from build123d import *

# Parameters (mm, degrees)
F0_W     = 2.35
F0_H     = 1.5
F1_DEPTH = 2.1
F2_START = -2.1
F0_R     = 2.8
F2_DEPTH = 0.9


with BuildPart() as f1:
    # F0 (on Right) → F1 (new body, symmetric)
    with BuildSketch(Plane.YZ):
        with BuildLine():
            Line((-3.65, 1.5), (-3.65, 2.1073284825))
            Line((-3.65, 2.1073284825), (0, 4.2146569651))
            Line((0, 4.2146569651), (3.65, 2.1073284825))
            Line((3.65, 2.1073284825), (3.65, -2.1073284825))
            Line((3.65, -2.1073284825), (0, -4.2146569651))
            Line((0, -4.2146569651), (-3.65, -2.1073284825))
            Line((-3.65, -2.1073284825), (-3.65, -1.5))
            Line((-3.65, -1.5), (-6, -1.5))
            Line((-6, -1.5), (-6, -5))
            Line((-6, -5), (6, -5))
            Line((6, -5), (6, 0))
            ThreePointArc((6, 0), (4.2426406871, 4.2426406871), (0, 6))
            ThreePointArc((0, 6), (-3.6742346142, 4.7434164903), (-5.8094750193, 1.5))
            Line((-5.8094750193, 1.5), (-3.65, 1.5))
        make_face()
        with Locations((-4.825, -0.75)):
            Rectangle(F0_W, F0_H)
        with BuildLine():
            Line((-3.65, 0), (-3.65, 1.5))
            Line((-3.65, 1.5), (-5.8094750193, 1.5))
            ThreePointArc((-5.8094750193, 1.5), (-5.9521781776, 0.7560257549), (-6, 0))
            Line((-6, 0), (-3.65, 0))
        make_face()
    extrude(amount=F1_DEPTH, both=True)

    # F0 (on Right) → F2 (join)
    with BuildSketch(Plane.YZ.offset(F2_START)):
        with BuildLine():
            Line((-3.65, 0), (-3.65, 1.5))
            Line((-3.65, 1.5), (-5.8094750193, 1.5))
            ThreePointArc((-5.8094750193, 1.5), (-5.9521781776, 0.7560257549), (-6, 0))
            Line((-6, 0), (-3.65, 0))
        make_face()
        with Locations((-4.825, -0.75)):
            Rectangle(F0_W, F0_H)
        with BuildLine():
            Line((-3.65, 1.5), (-3.65, 2.1073284825))
            Line((-3.65, 2.1073284825), (0, 4.2146569651))
            Line((0, 4.2146569651), (3.65, 2.1073284825))
            Line((3.65, 2.1073284825), (3.65, -2.1073284825))
            Line((3.65, -2.1073284825), (0, -4.2146569651))
            Line((0, -4.2146569651), (-3.65, -2.1073284825))
            Line((-3.65, -2.1073284825), (-3.65, -1.5))
            Line((-3.65, -1.5), (-6, -1.5))
            Line((-6, -1.5), (-6, -5))
            Line((-6, -5), (6, -5))
            Line((6, -5), (6, 0))
            ThreePointArc((6, 0), (4.2426406871, 4.2426406871), (0, 6))
            ThreePointArc((0, 6), (-3.6742346142, 4.7434164903), (-5.8094750193, 1.5))
            Line((-5.8094750193, 1.5), (-3.65, 1.5))
        make_face()
        Polygon((0, 4.2146569651), (-3.65, 2.1073284825), (-3.65, 1.5), (-3.65, 0), (-3.65, -1.5), (-3.65, -2.1073284825), (0, -4.2146569651), (3.65, -2.1073284825), (3.65, 2.1073284825), align=None)
        Circle(F0_R, mode=Mode.SUBTRACT)
    extrude(amount=-F2_DEPTH)

    # F0 (on Right) → F3 (revolve)
    with BuildSketch(Plane.YZ):
        with BuildLine():
            ThreePointArc((-6, 0), (-5.9521781776, 0.7560257549), (-5.8094750193, 1.5))
            Line((-5.8094750193, 1.5), (-13.15, 1.5))
            Line((-13.15, 1.5), (-13.15, 0))
            Line((-13.15, 0), (-6, 0))
        make_face()
        with BuildLine():
            Line((-3.65, 0), (-3.65, 1.5))
            Line((-3.65, 1.5), (-5.8094750193, 1.5))
            ThreePointArc((-5.8094750193, 1.5), (-5.9521781776, 0.7560257549), (-6, 0))
            Line((-6, 0), (-3.65, 0))
        make_face()
    revolve(axis=Axis((0, -8.4, 0), (0, 1, 0)))

    # F4: F1 across plane


with BuildPart() as f1_1:
    add(f1.part)
    add(f1.part.mirror(Plane.YZ))


solid = f1_1.part
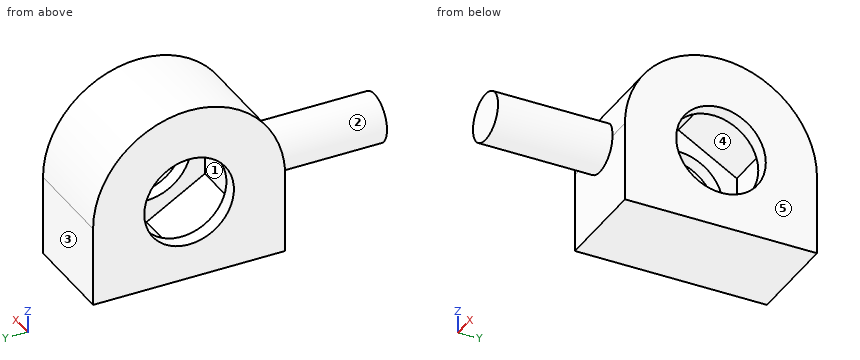
For this review, take the finished solid that the model builds, in its own axes (mm). Face numbers are marked on the shaded views. A direction names the side the tool comes from. Give positions to 0.01 mm unless a question says otherwise; leave off trailing zeros. Loops run counter-clockwise (first coordinate to the right, second up) from the corner with the lowest first, then second, coordinate; pieces in that order, holes last.
Item 1: Draft analysis for pull direction Y (two halves, no side actions). For the marked faces 1, 2 and 3, state which applies: +Y half, -Y half, draft (parallel to the pull), parting line (faces both ways), or undercut.
Item 2: For line 1 along Z through (x, y) = (2.8, 0); line 2 along X through (y, z) = (-2, 2); line 3 along Z through (x, y) = (0, -10.5), list the stretches that pass through material, from the lowest coordinate up.
Item 3: Take a section at B-B, the plane x = 0. State the section outline as (y, z) points.
Item 4: Take a section at D-D, the plane z = 4. State the section outline as (x, y) points.
Item 5: Take a section at C-C, the plane z = -2.5. State the section outline as (x, y) points, and give its area (3 significant figures).
Item 6: Take a section at A-A, the plane y = 1. State the section outline as (x, z) points, and give its area (3 significant figures).
Item 7: Tool access review of the marked faces 4 and 5: name each direction out of +Z, -Z, +X, -X, +Y, -Y from which nothing blocks a thin tool from reaching the whole face with its end or side.
Item 8: Insertion check: pin 1 (1 mm diameter, centred on x = -1, z = 5, fed in from +Y). The pin has a flat end and moves straight along its axis. Give the tip position at first contact, or say it passes through.
Calculated:
1. face 1: undercut
1. face 2: draft
1. face 3: +Y half
2. line 1: z = -5 to -2.8, 2.8 to 6
2. line 2: x = -3 to -2.1, 2.1 to 3
2. line 3: z = -1.5 to 1.5
3. outline: (-13.15, -1.5) - (-6, -1.5) - (-6, -5) - (6, -5) - (6, 0) arc R6 ccw to (-5.81, 1.5) - (-13.15, 1.5) - close; hole (-3.65, -2.11) - (0, -4.21) - (3.65, -2.11) - (3.65, 2.11) - (0, 4.21) - (-3.65, 2.11) - close
4. outline: (-3, -4.47) - (3, -4.47) - (3, 4.47) - (-3, 4.47) - close; hole (-2.1, -0.37) - (2.1, -0.37) - (2.1, 0.37) - (-2.1, 0.37) - close
5. outline: (-3, -6) - (3, -6) - (3, -1.26) - (2.1, -1.26) - (2.1, -2.97) - (-2.1, -2.97) - (-2.1, -1.26) - (-3, -1.26) - close; (-3, 1.26) - (-2.1, 1.26) - (-2.1, 2.97) - (2.1, 2.97) - (2.1, 1.26) - (3, 1.26) - (3, 6) - (-3, 6) - close
5. area: 42.5 mm2
6. outline: (-3, -5) - (3, -5) - (3, -2.62) - (2.1, -2.62) - (2.1, -3.64) - (-2.1, -3.64) - (-2.1, -2.62) - (-3, -2.62) - close; (-3, 2.62) - (-2.1, 2.62) - (-2.1, 3.64) - (2.1, 3.64) - (2.1, 2.62) - (3, 2.62) - (3, 5.92) - (-3, 5.92) - close
6. area: 25.5 mm2
7. face 4: none
7. face 5: +Z, -Z, +X, +Y, -Y
8. pin 1: stops at y = 3.97
